Model file for the job. Use its own axes, mm. Coordinates: 2 decimals unless noted, no trailing zeros. Write each loop counter-clockwise with the first axis right and the second up, starting at its lowest first coordinate (ties: lowest second). Pieces come first, ordered by that corner, then holes. Notation, with made-up numbers: (63, -30.75) - (73, -30.75) arc R15 ccw to (73, -17.75) - close; hole circle Ø6 at (57.25, 59). An arc over 180 degrees is marked (long way). Put each result on its own line as item: value. Start each with the question number.
1. Drill centre lines: L1, parallel to X at y = 15.5, z = 0.45; L2, parallel to X at y = 4.5, z = 1.1; L3, parallel to X at y = 10.75, z = 1.75. Where is each one in solid material? Low to high. Write a range as from..to.
2. Saw through at C-C, the plane x = 56. Write the cut outline in (y, z), plus the area to 3 significant figures.
3. Saw through at B-B, the plane y = 7.75. Write the cut outline in (x, z), plus the area to 3 significant figures.
4. Drop flat-ended pins along their axis: P1, Ø1.4, axis at x = -16.5, z = 1, coming from the +Y side; P2, Ø1.4, axis at y = 5, z = 1.5, coming from the -X side; P3, Ø0.8, axis at x = 88.5, z = 2, coming from the -Y side. Give the stop position or say it passes through.
5. Saw through at D-D, the plane x = 11.5. Write the cut outline in (y, z).
```python
from build123d import *

# Parameters (mm, degrees)
BOSS_EXTRUDE1_DEPTH = 2.794
FILLET1_R           = 2.54
SKETCH2_W           = 2.794
SKETCH2_H           = 12.7
SKETCH2_H_2         = 6.35
CUT_EXTRUDE1_DEPTH  = 99.618096392
FILLET2_R           = 12.7


with BuildPart() as part:
    # Sketch1 → Boss-Extrude1 (new body)
    with BuildSketch(Plane.XY):
        Polygon((0, 0), (95.25, 0), (95.25, 25.4), (82.55, 25.4), (82.55, 12.7), (12.7, 12.7), (12.7, 25.4), (0, 25.4), (0, 12.7), (-38.1, 12.7), (-38.1, 25.4), (-44.45, 25.4), (-44.45, 0), align=None)
    extrude(amount=BOSS_EXTRUDE1_DEPTH)

    # Fillet1
    fillet1_edges = [part.edges().sort_by_distance(p)[0] for p in [
        (-44.45, 25.4, 1.397),
        (-38.1, 25.4, 1.397),
        (-38.1, 12.7, 1.397),
        (0, 12.7, 1.397),
        (0, 25.4, 1.397),
        (12.7, 25.4, 1.397),
        (82.55, 25.4, 1.397),
        (95.25, 25.4, 1.397),
        (95.25, 0, 1.397),
    ]]
    fillet(fillet1_edges, radius=FILLET1_R)

    # Sketch2 → Cut-Extrude1 (cut, through all)
    with BuildSketch(Plane.XY.offset(2.794)):
        with Locations((89.115859958, 6.35)):
            Rectangle(SKETCH2_W, SKETCH2_H)
        with Locations((6.946859958, 6.35)):
            Rectangle(SKETCH2_W, SKETCH2_H)
        with Locations((68.453, 9.525)):
            Rectangle(SKETCH2_W, SKETCH2_H_2)
    extrude(amount=-CUT_EXTRUDE1_DEPTH, mode=Mode.SUBTRACT)

    # Fillet2
    fillet2_edges = [part.edges().sort_by_distance(p)[0] for p in [
        (-44.45, 0, 1.397),
    ]]
    fillet(fillet2_edges, radius=FILLET2_R)


solid = part.part
```
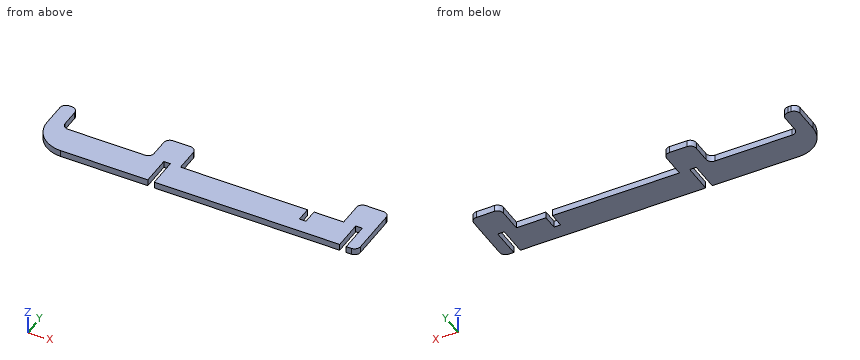
Final values:
1. L1: x = -44.45..-38.1, 0..12.7, 82.55..95.25
1. L2: x = -41.45..5.55, 8.34..87.72, 90.51..95.25
1. L3: x = -44.3..5.55, 8.34..67.06, 69.85..87.72, 90.51..95.25
2. outline: (0, 0) - (12.7, 0) - (12.7, 2.79) - (0, 2.79) - close
2. area: 35.5 mm²
3. outline: (-43.45, 0) - (5.55, 0) - (5.55, 2.79) - (-43.45, 2.79) - close; (8.34, 0) - (67.06, 0) - (67.06, 2.79) - (8.34, 2.79) - close; (69.85, 0) - (87.72, 0) - (87.72, 2.79) - (69.85, 2.79) - close; (90.51, 0) - (95.25, 0) - (95.25, 2.79) - (90.51, 2.79) - close
3. area: 364 mm²
4. P1: stops at y = 12.7
4. P2: stops at x = -42.35
4. P3: stops at y = 12.7
5. outline: (0, 0) - (25.02, 0) - (25.02, 2.79) - (0, 2.79) - close
